Design review of the part built by this model. Coordinates are the model's own, in mm. A direction names the side the tool comes from. Give positions to 0.01 mm unless a question says otherwise; leave off trailing zeros. Write each loop counter-clockwise with the first axis right and the second up, starting at its lowest first coordinate (ties: lowest second). Pieces come first, ordered by that corner, then holes. Notation, with made-up numbers: (-31.5, 31) - (-11.5, 31) arc R14 ccw to (-11.5, 39) - close; hole circle Ø8 at (24, 66.25). An arc over 180 degrees is marked (long way). Use a Markdown table: item, result. Add a question column.
Autodesk Inventor part; units mm, degrees
ref_plane "bolt_XY" through (0, 0, 0) normal (1, 0, 0) x (0, 0, -1)
ref_plane "bolt_YZ" through (0, 0, 0) normal (0, 0, -1) x (0, 1, 0)
ref_plane "bolt_ZX" through (0, 0, 0) normal (0, 1, 0) x (1, 0, 0)
sketch "Sketch_1" plane through (0, 0, 0) normal (0, 0, 1) x (1, 0, 0)
  line L0 (6, 0) -> (-1.6, 0)
  line L1 (-1.6, 0) -> (-1.6, 2.25)
  line L2 (-1.6, 2.25) -> (0, 2.25)
  line L3 (0, 2.25) -> (0, 1.35)
  arc A0 (0, 1.35) -> (0.1, 1.25) centre (0.1, 1.35) ccw
  line L4 (0.1, 1.25) -> (5.724, 1.25)
  line L5 (5.724, 1.25) -> (6, 0.974)
  line L6 (6, 0.974) -> (6, 0)
  line L7 (6, 0) -> (-1.6, 0)
revolve "Revolution1" add sketch "Sketch_1" angle 360 about axis through (6, 0, 0) along (1, 0, 0)
thread "Thread1"
sketch "Sketch2" plane through (-1.6, 0, 0) normal (-1, 0, 0) x (0, 0, 1)
  point P0 (0, 0)
hole "Hole1" at (-1.6, 0, 0) direction (1, 0, 0) diameter 1.5 depth 1.3 tip angle 140
sketch "Sketch_3" plane through (-1.6, 0, 0) normal (1, 0, 0) x (0, 0, -1)
  line L0 (-0.75, -0.433) -> (0, -0.866)
  line L1 (0, -0.866) -> (0.75, -0.433)
  line L2 (0.75, -0.433) -> (0.75, 0.433)
  line L3 (0.75, 0.433) -> (0, 0.866)
  line L4 (0, 0.866) -> (-0.75, 0.433)
  line L5 (-0.75, 0.433) -> (-0.75, -0.433)
extrude "Extrusion1" cut sketch "Sketch_3" along normal blind 1.3
ref_plane "bolt_XY" through (0, 0, 0) normal (1, 0, 0) x (0, 0, -1)
ref_plane "bolt_YZ" through (0, 0, 0) normal (0, 0, -1) x (0, 1, 0)
ref_plane "bolt_ZX" through (0, 0, 0) normal (0, 1, 0) x (1, 0, 0)
ref_plane "bolt_to_nut_XY" through (6, 0, 0) normal (1, 0, 0) x (0, 0, -1)
ref_plane "bolt_to_nut_YZ" through (6, 0, 0) normal (0, 0, -1) x (0, 1, 0)
ref_plane "bolt_to_nut_ZX" through (6, 0, 0) normal (0, 1, 0) x (1, 0, 0)
properties part number "CBSST2_5-6"
(1) For line 1 along Z through (x, y) = (0.5, 1); line 2 along Y through (x, z) = (5.25, 0.05); line 3 along X through (y, z) = (1.3, 0.85), list the stretches that pass through material, from the lowest coordinate up.
(2) Add section B-B (z = -1.65). State the section outline as (x, y) points, and give its area (3 significant figures).
(3) Insertion check: pin 1 (2 mm diameter, centred on y = -1.5, z = 1.5, fed in from +X); pin 2 (1 mm diameter, centred on x = 5, y = -1.5, fed in from +Z). Each pin has a flat end and moves straight along its axis. Give the tip position at first contact, or say it passes through.
(4) Tool access review of faces 4 (the face through (-0.79, -0.29, 2.23)), 5 (the face through (-1, 0, 0.75)): name each direction out of +Z, -Z, +X, -X, +Y, -Y from which nothing blocks a thin tool from reaching the whole face with its end or side.
(5) Mouldability with a two-part tool opening along Y and no side actions: class faces 1 (the face through (-1, 0, -0.75)), 2 (the face through (0, 0.5, -1.5)), 3 (the face through (2.95, -0.27, -1.22)) as +Y half, -Y half, draft (parallel to the pull), parting line (faces both ways), or undercut.
(6) Add section A-A (x = 1.75). State the section outline as (y, z) points.
Answers follow:
| question | item | result |
|---|---|---|
| 1 | line 1 | -0.75 to 0.75 |
| 1 | line 2 | -1.25 to 1.25 |
| 1 | line 3 | -1.6 to 0 |
| 2 | outline | (-1.6, -1.53) - (0, -1.53) - (0, 1.53) - (-1.6, 1.53) - close |
| 2 | area | 4.90 mm^2 |
| 3 | pin 1 | x = 5.85 |
| 3 | pin 2 | z = 0.75 |
| 4 | face 4 | +X, -X |
| 4 | face 5 | -X |
| 5 | face 1 | undercut |
| 5 | face 2 | draft |
| 5 | face 3 | parting line |
| 6 | outline | circle Ø2.5 at (0, 0) |
